Geometry check sheet. Reference: the model listing, model coordinates, mm. Give positions to 0.01 mm unless a question says otherwise; leave off trailing zeros. Loops run counter-clockwise (first coordinate to the right, second up) from the corner with the lowest first, then second, coordinate; pieces in that order, holes last.
1. Material ranges on L1, parallel to Z at x = 15.5, y = 6; L2, parallel to X at y = 11.5, z = -15; L3, parallel to X at y = 3.75, z = 17, recorded low to high.
2. Cross-section at B-B, the plane x = -15.5. Record the cut outline in (y, z).
3. Cross-section at C-C, the plane y = 4. Record the cut outline in (x, z), plus the area to 3 significant figures.
4. Cross-section at A-A, the plane z = 0. Record the cut outline in (x, y), plus the area to 3 significant figures.
5. Release check for a two-part mould opening along X. For faces 1 (the flat face through (-9, 0, 0)), 2 (the flat face through (-20, 6, 0)), 3 (the cylindrical face through (14.6, 6.3, 14)) record: +X half, -X half, draft (parallel to the pull), parting line (faces both ways), or undercut.
6. Go/stop test with flat-tipped pins: pin 1 Ø4 at (x, z) = (-4.5, -2) entering from +Y; pin 2 Ø8 at (x, z) = (0.5, 1) entering from -Y. Record where each tip stops, or that it passes through.
7. Cross-section at D-D, the plane z = -15.5. Record the cut outline in (x, y), plus the area to 3 significant figures.
Autodesk Inventor part; units mm, degrees
ref_plane "YZ Plane" through (0, 0, 0) normal (1, 0, 0) x (0, 1, 0)
ref_plane "XZ Plane" through (0, 0, 0) normal (0, 1, 0) x (-1, 0, 0)
ref_plane "XY Plane" through (0, 0, 0) normal (0, 0, 1) x (1, 0, 0)
sketch "Sketch1" plane through (0, 0, 0) normal (0, 1, 0) x (-1, 0, 0)
  line L0 (-20, -20) -> (20, -20)
  line L1 (20, -20) -> (20, 20)
  line L2 (20, 20) -> (-20, 20)
  line L3 (-20, 20) -> (-20, -20)
  line L4 (-20, -20) -> (20, 20) construction
  line L5 (20, -20) -> (-20, 20) construction
  circle A0 centre (15.5, 15.5) radius 1.75
  line L6 (20, 0) -> (-20, 0)
  line L7 (0, -20) -> (0, 20)
  circle A1 centre (15.5, -15.5) radius 1.75
  circle A2 centre (-15.5, 15.5) radius 1.75
  circle A3 centre (-15.5, -15.5) radius 1.75
  point P0 (0, 0)
  dimension "d3" = 40
  dimension "d4" = 40
  dimension "d5" = 3.5
  dimension "d10" = 31
  dimension "d11" = 31
extrude "Extrusion2" add sketch "Sketch1" along normal blind 12.7
sketch "Sketch2" plane through (0, 0, 0) normal (0, -1, 0) x (1, 0, 0)
  circle A0 centre (0, 0) radius 6.75
  dimension "d12" = 13.5
extrude "Extrusion3" cut sketch "Sketch2" against normal through all
properties part number "Lead_Screw_Thrust_Bearing_Mount"
Result:
1. L1: z = -20 to -17.25, -13.75 to 13.75, 17.25 to 20
1. L2: x = -20 to -17.18, -13.82 to 13.82, 17.18 to 20
1. L3: x = -20 to -16.4, -14.6 to 14.6, 16.4 to 20
2. outline: (0, -20) - (12.7, -20) - (12.7, -17.25) - (0, -17.25) - close; (0, -13.75) - (12.7, -13.75) - (12.7, 13.75) - (0, 13.75) - close; (0, 17.25) - (12.7, 17.25) - (12.7, 20) - (0, 20) - close
3. outline: (-20, -20) - (20, -20) - (20, 20) - (-20, 20) - close; hole circle Ø3.5 at (-15.5, -15.5); hole circle Ø3.5 at (-15.5, 15.5); hole circle Ø13.5 at (0, 0); hole circle Ø3.5 at (15.5, -15.5); hole circle Ø3.5 at (15.5, 15.5)
3. area: 1,420 mm2
4. outline: (-20, 0) - (-6.75, 0) - (-6.75, 12.7) - (-20, 12.7) - close; (6.75, 0) - (20, 0) - (20, 12.7) - (6.75, 12.7) - close
4. area: 337 mm2
5. face 1: draft
5. face 2: -X half
5. face 3: undercut
6. pin 1: stops at y = 12.7
6. pin 2: passes through
7. outline: (-20, 0) - (-17.25, 0) - (-17.25, 12.7) - (-20, 12.7) - close; (-13.75, 0) - (13.75, 0) - (13.75, 12.7) - (-13.75, 12.7) - close; (17.25, 0) - (20, 0) - (20, 12.7) - (17.25, 12.7) - close
7. area: 419 mm2
